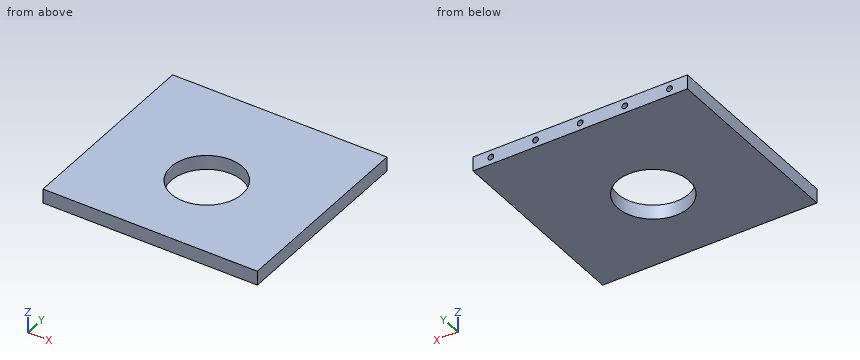
from build123d import *

# Parameters (mm, degrees)
SKETCH1_W                              = 120
SKETCH1_H                              = 110
BOSS_EXTRUDE1_DEPTH                    = 8
TAP_DRILL_FOR_M3_HELICOIL1_D           = 3.15
TAP_DRILL_FOR_M3_HELICOIL1_DEPTH       = 6
TAP_DRILL_FOR_M3_HELICOIL1_CSINK_D     = 3.2
TAP_DRILL_FOR_M3_HELICOIL1_CSINK_ANGLE = 90
TAP_DRILL_FOR_M3_HELICOIL1_TIP         = 0.946355475
F_40_0_40_DIAMETER_HOLE1_D             = 40


with BuildPart() as part:
    # Sketch1 → Boss-Extrude1 (new body)
    with BuildSketch(Plane.XY):
        with Locations((60, 55)):
            Rectangle(SKETCH1_W, SKETCH1_H)
    extrude(amount=BOSS_EXTRUDE1_DEPTH)

    # Tap Drill for M3 Helicoil1
    with Locations(Plane(origin=(0, 110, 0), x_dir=(1, 0, 0), z_dir=(0, 1, 0))):
        with Locations((10, -4), (60, -4), (85, -4), (110, -4), (35, -4)):
            CounterSinkHole(TAP_DRILL_FOR_M3_HELICOIL1_D / 2, TAP_DRILL_FOR_M3_HELICOIL1_CSINK_D / 2, depth=TAP_DRILL_FOR_M3_HELICOIL1_DEPTH, counter_sink_angle=TAP_DRILL_FOR_M3_HELICOIL1_CSINK_ANGLE)
            with Locations((0, 0, -(TAP_DRILL_FOR_M3_HELICOIL1_DEPTH + TAP_DRILL_FOR_M3_HELICOIL1_TIP / 2))):  # 118° drill point
                Cone(0, TAP_DRILL_FOR_M3_HELICOIL1_D / 2, TAP_DRILL_FOR_M3_HELICOIL1_TIP, mode=Mode.SUBTRACT)

    # Ø40.0 (40) Diameter Hole1 (through all)
    with Locations(Plane(origin=(0, 0, 0), x_dir=(-1, 0, 0), z_dir=(0, 0, -1))):
        with Locations((-60, 48)):
            Hole(F_40_0_40_DIAMETER_HOLE1_D / 2)


solid = part.part
Model file for the job. Use its own axes, mm. Round coordinates to 2 decimals unless told otherwise and drop trailing zeros. Loops run counter-clockwise (first coordinate to the right, second up) from the corner with the lowest first, then second, coordinate; pieces in that order, holes last.
1. Band-saw the part on A-A, the plane y = 57. List the corners of the cut face in (x, z).
Check values:
outline: (0, 0) - (42.14, 0) - (42.14, 8) - (0, 8) - close; (77.86, 0) - (120, 0) - (120, 8) - (77.86, 8) - close
2. Drop a flat-ended pin along its axis: P1, Ø1.9, axis at x = 60, z = 4, coming from the +Y side. Give the stop position or say it passes through.
Check values:
P1: stops at y = 103.62
3. Band-saw the part on B-B, the plane x = 44.5. List the corners of the cut face in (y, z), and give its area (3 significant figures).
Check values:
outline: (0, 0) - (35.36, 0) - (35.36, 8) - (0, 8) - close; (60.64, 0) - (110, 0) - (110, 8) - (60.64, 8) - close
area: 678 mm2
4. Wall check: probe 1 along X at (y, z) = (106.1, 4) (3 decimals); probe 2 along Z at (x, y) = (10, 106.8) (3 decimals); probe 3 along Y at (x, z) = (60, 6.25). Give the ranges that are in metal, low to high.
Check values:
probe 1: x = 0 to 8.425, 11.575 to 33.425, 36.575 to 58.425, 61.575 to 83.425, 86.575 to 108.425, 111.575 to 120
probe 2: z = 0 to 2.425, 5.575 to 8
probe 3: y = 0 to 28, 68 to 110
